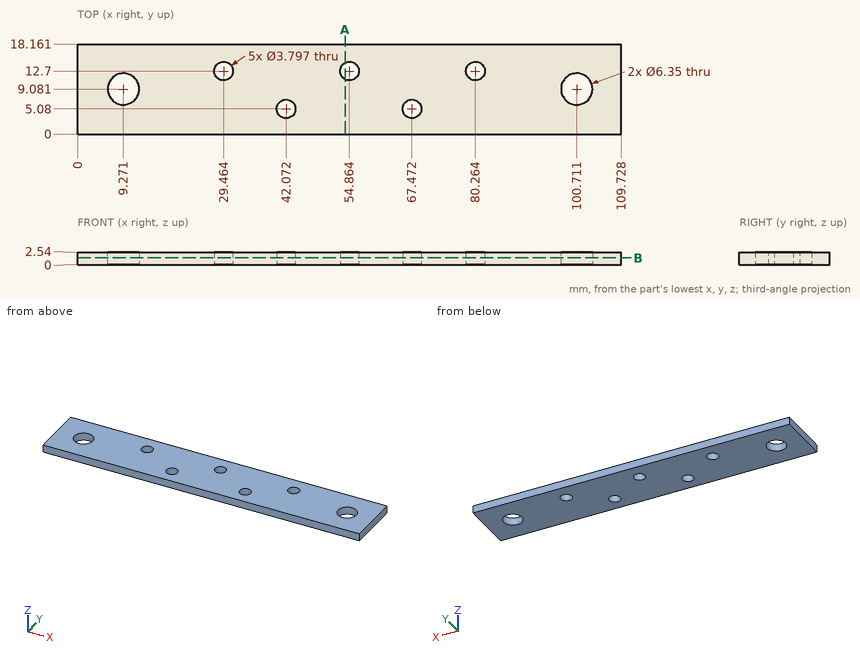
Can you work these out from the drawing? Everything is in mm from the part's minimum corner. Round coordinates to 2 decimals unless told otherwise and drop trailing zeros. Order: outer loops, then holes, each group sorted by start corner. A loop starts at its lowest first (then second) coordinate and runs counter-clockwise, first axis right, second up. Notation, with made-up numbers: (-1, 1) - (53, 1) arc R23 ccw to (53, 28) - close; hole circle Ø9 at (55.25, 29). An arc over 180 degrees is marked (long way). Answer in a Markdown table with one row per item.
(1) Suppose I cut it at A-A, the plane x = 54. Please give me the cut outline in (y, z).
From the geometry:
| item | result |
|---|---|
| outline | (0, 0) - (11.01, 0) - (11.01, 2.54) - (0, 2.54) - close; (14.39, 0) - (18.16, 0) - (18.16, 2.54) - (14.39, 2.54) - close |
(2) Please list where these lines run through material, in increasing order: L1, parallel to X at y = 12.75, z = 0.25 (1 decimal); L2, parallel to X at y = 9, z = 2.15 (1 decimal); L3, parallel to X at y = 14.25, z = 2.15 (1 decimal). Write a range as from..to.
From the geometry:
| item | result |
|---|---|
| L1 | x = 0..27.6, 31.4..53, 56.8..78.4, 82.2..109.7 |
| L2 | x = 0..6.1, 12.4..97.5, 103.9..109.7 |
| L3 | x = 0..28.4, 30.6..53.8, 56..79.2, 81.4..109.7 |
(3) For P1, Ø5, axis at x = 80.264, y = 12.7, coming from the +Z side, with a flat end and sliding along its axis, tell me the tip position at first contact or that it passes through.
From the geometry:
| item | result |
|---|---|
| P1 | stops at z = 2.54 |
(4) Suppose I cut it at B-B, the plane z = 1.35. Count the separate pieces of the cut face and the enclosed holes in it, plus the area to 3 significant figures.
From the geometry:
| item | result |
|---|---|
| separate pieces | 1 |
| enclosed holes | 7 |
| area | 1,870 mm2 |
